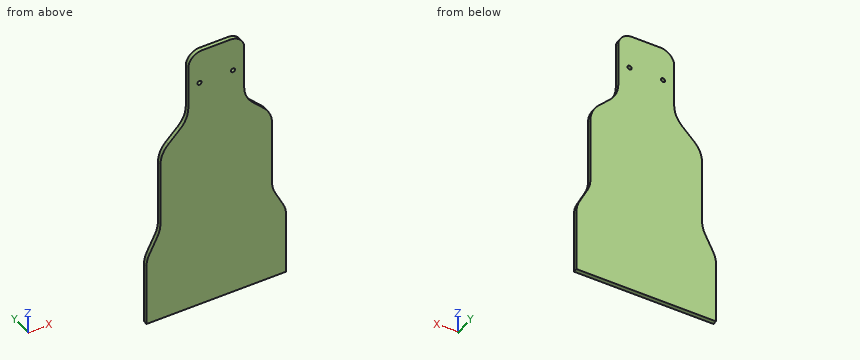
Autodesk Inventor part; units mm, degrees
ref_plane "Work Plane1" through (0, 0, -25) normal (0, 0, 1) x (1, 0, 0)
ref_plane "YZ Plane" through (0, 0, 0) normal (1, 0, 0) x (0, 1, 0)
ref_plane "XZ Plane" through (0, 0, 0) normal (0, 1, 0) x (-1, 0, 0)
sketch "Sketch1" plane through (0, 0, 0) normal (0, 1, 0) x (-1, 0, 0)
  line L0 (0, -154.7214) -> (0, -200)
  line L1 (0, -200) -> (-100, -200)
  line L2 (-100, -200) -> (-100, -154.7214)
  line L3 (-60, 0) -> (-40, 0)
  line L4 (-2.1115, -145.7771) -> (-7.8885, -134.2229)
  line L5 (-10, -125.2786) -> (-10, -78.2843)
  line L6 (-15.8579, -64.1421) -> (-24.1421, -55.8579)
  line L7 (-30, -41.7157) -> (-30, -10)
  line L8 (-70, -10) -> (-70, -41.7157)
  line L9 (-75.8579, -55.8579) -> (-84.1421, -64.1421)
  line L10 (-90, -78.2843) -> (-90, -125.2786)
  line L11 (-92.1115, -134.2229) -> (-97.8885, -145.7771)
  arc A0 (-30, -41.7157) -> (-24.1421, -55.8579) centre (-10, -41.7157) ccw
  arc A1 (-75.8579, -55.8579) -> (-70, -41.7157) centre (-90, -41.7157) ccw
  arc A2 (-84.1421, -64.1421) -> (-90, -78.2843) centre (-70, -78.2843) ccw
  arc A3 (-10, -78.2843) -> (-15.8579, -64.1421) centre (-30, -78.2843) ccw
  arc A4 (-10, -125.2786) -> (-7.8885, -134.2229) centre (10, -125.2786) ccw
  arc A5 (-92.1115, -134.2229) -> (-90, -125.2786) centre (-110, -125.2786) ccw
  arc A6 (-97.8885, -145.7771) -> (-100, -154.7214) centre (-80, -154.7214) ccw
  arc A7 (0, -154.7214) -> (-2.1115, -145.7771) centre (-20, -154.7214) ccw
  arc A8 (-30, -10) -> (-40, 0) centre (-40, -10) ccw
  arc A9 (-60, 0) -> (-70, -10) centre (-60, -10) ccw
  point P0 (0, 0)
  point P1 (-100, 0)
  point P2 (0, -150)
  point P3 (-10, -130)
  point P4 (-10, -70)
  point P5 (-30, -50)
  point P6 (-30, 0)
  point P7 (-70, 0)
  point P8 (-70, -50)
  point P9 (-90, -70)
  point P10 (-90, -130)
  point P11 (-100, -150)
  point P12 (0, 0)
  dimension "d23" = 50
  dimension "d24" = 60
  dimension "d25" = 60
  dimension "d26" = 50
  dimension "d27" = 50
  dimension "d28" = 50
  dimension "d29" = 20
  dimension "d30" = 20
  dimension "d31" = 40
  dimension "d32" = 100
  dimension "d34" = 10
  dimension "d35" = 10
  dimension "d36" = 20
  dimension "d37" = 200
  dimension "d38" = 20
  dimension "d39" = 10
extrude "Extrusion2" add sketch "Sketch1" against normal blind 3
ref_plane "Work Plane1" through (0, 0, -25) normal (0, 0, 1) x (1, 0, 0)
sketch "Sketch8" plane through (0, 0, 0) normal (0, 1, 0) x (1, 0, 0)
  line L0 (70, 10) -> (70, 41.7157)
  line L1 (30, 41.7157) -> (30, 10)
  line L2 (40, 0) -> (60, 0)
  point P0 (0, 0)
  point P1 (38, 25)
  point P2 (62, 25)
  dimension "d117" = 8
  dimension "d118" = 8
  dimension "d119" = 25
  dimension "d120" = 25
hole "Hole2" at (38, 0, -25) at (62, 0, -25) direction (0, -1, 0) diameter 3 end through all
thread "Thread1"
thread "Thread2"
properties part number "base_plate" material "Acrylic, Clear"
Read the model definition and answer for the solid it produces. Units are mm, in the model's axes. Give positions to 0.01 mm unless a question says otherwise; leave off trailing zeros. Order: outer loops, then holes, each group sorted by start corner. A loop starts at its lowest first (then second) coordinate and runs counter-clockwise, first axis right, second up. Notation, with made-up numbers: (20, 37) -> (64, 37) arc R5 ccw to (64, 46) -> close; hole circle Ø10 at (-21, 87.25). An arc over 180 degrees is marked (long way). One line per item, written item: value. Start each with the question number.
(1) Straight lines are drawn through the part: L1, parallel to X at y = -1.65, z = -25; L2, parallel to X at y = -0.35, z = -36.5; L3, parallel to Z at x = 37, y = -2.65. For each, find the intervals that lie inside material, in ascending order.
(2) Flat-ended cylindrical pins translate along their axes: P1, Ø1.5, axis at y = -1, z = -105, coming from the -X side; P2, Ø3, axis at x = 42.5, z = -30.5, coming from the +Y side; P3, Ø0.9, axis at y = -1, z = -28, coming from the +X side. Find the tip coordinate at first contact, or state that the pin passes through.
(3) The part is cut by section A-A (y = -1.5). Determine the outline of the cut face in (x, z).
(4) The part is cut by section B-B (x = 82). Determine the outline of the cut face in (y, z), and give its area (3 significant figures).
(5) The part is cut by section C-C (z = -29). Determine the outline of the cut face in (x, y).
Taken from the geometry:
1. L1: 30 to 36.5, 39.5 to 60.5, 63.5 to 70
1. L2: 30 to 70
1. L3: -200 to -26.12, -23.88 to -0.46
2. P1: x = 10
2. P2: y = 0
2. P3: x = 70
3. outline: (0, -200) -> (100, -200) -> (100, -154.72) arc R20 ccw to (97.89, -145.78) -> (92.11, -134.22) arc R20 cw to (90, -125.28) -> (90, -78.28) arc R20 ccw to (84.14, -64.14) -> (75.86, -55.86) arc R20 cw to (70, -41.72) -> (70, -10) arc R10 ccw to (60, 0) -> (40, 0) arc R10 ccw to (30, -10) -> (30, -41.72) arc R20 cw to (24.14, -55.86) -> (15.86, -64.14) arc R20 ccw to (10, -78.28) -> (10, -125.28) arc R20 cw to (7.89, -134.22) -> (2.11, -145.78) arc R20 ccw to (0, -154.72) -> close; hole circle Ø3 at (38, -25); hole circle Ø3 at (62, -25)
4. outline: (-3, -200) -> (0, -200) -> (0, -62) -> (-3, -62) -> close
4. area: 414 mm^2
5. outline: (30, -3) -> (70, -3) -> (70, 0) -> (30, 0) -> close
